The listing builds one solid part. Answer for the finished solid, in the listing's coordinates (mm). A direction names the side the tool comes from. Coordinates: 2 decimals unless noted, no trailing zeros. Write each loop counter-clockwise with the first axis right and the second up, starting at its lowest first coordinate (ties: lowest second). Pieces come first, ordered by that corner, then holes.
(1) The part is cut by section B-B on z = 9.75. Determine the outline of the cut face in (x, y), plus the area to 3 significant figures.
(2) Straight lines are drawn through the part: line 1 (X direction, y = 17.3, z = 3.75); line 2 (X direction, y = -1.5, z = 3.75); line 3 (Y direction, x = -2, z = 9). For each, find the intervals that lie inside material, in ascending order.
(3) For a pull along Y with two mould halves and no side action, classify faces 4 (the flat face through (0, 28.8, 1)), 5 (the flat face through (-7.1, -1, 9)), 6 (the flat face through (-8.5, 1, 6)) as +Y half, -Y half, draft (parallel to the pull), parting line (faces both ways), or undercut.
(4) The part is cut by section D-D on x = -6.5. Determine the outline of the cut face in (y, z), plus the area to 3 significant figures.
(5) The part is cut by section C-C on y = -30. Determine the outline of the cut face in (x, z), plus the area to 3 significant figures.
(6) The part is cut by section A-A on y = 17.3. Determine the outline of the cut face in (x, z), plus the area to 3 significant figures.
(7) Given P1, Ø4, axis at x = -4, y = -11.5, coming from the -Z side; P2, Ø1, axis at x = 2.5, z = 8, coming from the +Y side; P3, Ø7, axis at x = 2, y = 10, coming from the +Z side; P4, Ø4, axis at x = -2, y = 32.5, coming from the +Z side, each flat-ended and moving along its own axis, determine where each tip first touches the part or whether it passes through.
(8) Which of the six approach directions +Z, -Z, +X, -X, +Y, -Y give full straight-line access (tool end or side, diameter ignored) to faces 1 (the flat face through (0, 28.8, 8)), 2 (the flat face through (-1.6, -28, 9)), 3 (the flat face through (0, 31, 1.4))?
from build123d import *

# Parameters (mm, degrees)
F0_W      = 17
F0_H      = 68
F1_DEPTH  = 11.3
F2_R      = 3
F4_DEPTH  = 5
F6_DEPTH  = 25
F7_W      = 10.167095
F7_H      = 8.266306
F7_H_2    = 5.37331
F8_DEPTH  = 25
F9_R      = 5
F10_DEPTH = 25


with BuildPart() as f1:
    # F0 (on Top) → F1 (new body)
    with BuildSketch(Plane.XY):
        Rectangle(F0_W, F0_H)
    extrude(amount=F1_DEPTH)

    # F2
    f2_edges = [f1.edges().sort_by_distance(p)[0] for p in [
        (8.5, -34, 5.65),
        (-8.5, -34, 5.65),
    ]]
    fillet(f2_edges, radius=F2_R)

    # F3 (on face) → F4 (cut)
    with BuildSketch(Plane.XY.offset(11.3)):
        with BuildLine():
            ThreePointArc((-7.1, -30.6), (-6.514214, -32.014214), (-5.1, -32.6))
            Line((-5.1, -32.6), (-1.6, -32.6))
            Line((-1.6, -32.6), (-1.6, -23.3))
            Line((-1.6, -23.3), (1.6, -23.3))
            Line((1.6, -23.3), (1.6, -32.6))
            Line((1.6, -32.6), (5.1, -32.6))
            ThreePointArc((5.1, -32.6), (6.514214, -32.014214), (7.1, -30.6))
            Line((7.1, -30.6), (7.1, 27.4))
            Line((7.1, 27.4), (-7.1, 27.4))
            Line((-7.1, 27.4), (-7.1, -30.6))
        make_face()
    extrude(amount=-F4_DEPTH, mode=Mode.SUBTRACT)

    # F5 (on face) → F6 (cut)
    with BuildSketch(Plane.XY.offset(6.3)):
        with BuildLine():
            ThreePointArc((0, -19.7), (2.12132, -18.82132), (3, -16.7))
            Line((3, -16.7), (3, 17.3))
            ThreePointArc((3, 17.3), (2.12132, 19.42132), (0, 20.3))
            ThreePointArc((0, 20.3), (-2.12132, 19.42132), (-3, 17.3))
            Line((-3, 17.3), (-3, -16.7))
            ThreePointArc((-3, -16.7), (-2.12132, -18.82132), (0, -19.7))
        make_face()
    extrude(amount=-F6_DEPTH, mode=Mode.SUBTRACT)

    # F7 (on face) → F8 (cut)
    with BuildSketch(Plane.YZ.offset(8.5)):
        with Locations((33.883547, 9.533153)):
            Rectangle(F7_W, F7_H)
        with Locations((33.883547, -1.286655)):
            Rectangle(F7_W, F7_H_2)
    extrude(amount=-F8_DEPTH, mode=Mode.SUBTRACT)

    # F9 (on face) → F10 (cut)
    with BuildSketch(Plane.XY.offset(6.3)):
        with Locations((0, 17.3)):
            Circle(F9_R)
    extrude(amount=-F10_DEPTH, mode=Mode.SUBTRACT)


solid = f1.part
Model answer:
1. outline: (-8.5, -31) arc R3 ccw to (-5.5, -34) - (5.5, -34) arc R3 ccw to (8.5, -31) - (8.5, 28.8) - (-8.5, 28.8) - close; hole (-7.1, -30.6) arc R2 ccw to (-5.1, -32.6) - (-1.6, -32.6) - (-1.6, -23.3) - (1.6, -23.3) - (1.6, -32.6) - (5.1, -32.6) arc R2 ccw to (7.1, -30.6) - (7.1, 27.4) - (-7.1, 27.4) - close
1. area: 243 mm2
2. line 1: x = -8.5 to -5, 5 to 8.5
2. line 2: x = -8.5 to -3, 3 to 8.5
2. line 3: y = -34 to -32.6, 27.4 to 28.8
3. face 4: +Y half
3. face 5: undercut
3. face 6: draft
4. outline: (-33.83, 0) - (28.8, 0) - (28.8, 1.4) - (34, 1.4) - (34, 5.4) - (28.8, 5.4) - (28.8, 11.3) - (27.4, 11.3) - (27.4, 6.3) - (-32.03, 6.3) - (-32.03, 11.3) - (-33.83, 11.3) - close
4. area: 431 mm2
5. outline: (-8.5, 0) - (8.5, 0) - (8.5, 11.3) - (7.1, 11.3) - (7.1, 6.3) - (1.6, 6.3) - (1.6, 11.3) - (-1.6, 11.3) - (-1.6, 6.3) - (-7.1, 6.3) - (-7.1, 11.3) - (-8.5, 11.3) - close
5. area: 137 mm2
6. outline: (-8.5, 0) - (-5, 0) - (-5, 6.3) - (-7.1, 6.3) - (-7.1, 11.3) - (-8.5, 11.3) - close; (5, 0) - (8.5, 0) - (8.5, 11.3) - (7.1, 11.3) - (7.1, 6.3) - (5, 6.3) - close
6. area: 58.1 mm2
7. P1: stops at z = 0
7. P2: stops at y = 28.8
7. P3: stops at z = 6.3
7. P4: stops at z = 5.4
8. face 1: +Z, +X, -X, +Y
8. face 2: +Z
8. face 3: -Z, +X, -X, +Y
